Geometry: final body of the model. Coordinates: model frame, mm. A direction names the side the tool comes from. Coordinates: 2 decimals unless noted, no trailing zeros. Loops run counter-clockwise (first coordinate to the right, second up) from the corner with the lowest first, then second, coordinate; pieces in that order, holes last. Notation, with made-up numbers: (31.5, 60.25) - (48.5, 60.25) arc R26 cw to (48.5, 83.25) - close; hole circle Ø3 at (76.25, 9.5). An arc over 180 degrees is marked (long way). Return JSON: item names as keys, results as strings.
from build123d import *

# Parameters (mm, degrees)
F0_W      = 5
F0_H      = 25.21445
F1_DEPTH  = 25
F2_DEPTH  = 25
F3_W      = 40.349028
F3_H      = 25.21445
F3_W_2    = 5
F4_DEPTH  = 25
F6_DEPTH  = 25
F7_W      = 19.362385
F7_H      = 69.068812
F8_DEPTH  = 22
F9_W      = 17.915649
F9_H      = 21.240922
F10_DEPTH = 40


with BuildPart() as f1:
    # F0 (on Front) → F1 (new body)
    with BuildSketch(Plane.XZ):
        Polygon((0, 50.428901), (0, 25.21445), (5, 25.21445), (5, 45.428901), (50.775229, 45.428901), (50.775229, 0), (55.775229, 0), (55.775229, 50.428901), align=None)
        with Locations((2.5, 12.607225)):
            Rectangle(F0_W, F0_H)
    extrude(amount=-F1_DEPTH)

    # F0 (on Front) → F2 (join)
    with BuildSketch(Plane.XZ):
        with Locations((2.5, 12.607225)):
            Rectangle(F0_W, F0_H)
    extrude(amount=F2_DEPTH)

    # F3 (on face) → F4 (join)
    with BuildSketch(Plane.XZ.offset(25)):
        with Locations((25.174514, 12.607225)):
            Rectangle(F3_W, F3_H)
        with Locations((2.5, 12.607225)):
            Rectangle(F3_W_2, F3_H)
    extrude(amount=F4_DEPTH)

    # F5 (on face) → F6 (join)
    with BuildSketch(Plane(origin=(0, 0, 0), x_dir=(0, -1, 0), z_dir=(-1, 0, 0))):
        Polygon((-25, 25.21445), (-25, 0), (50, 0), (50, 25.21445), (0, 25.21445), align=None)
    extrude(amount=F6_DEPTH)

    # F7 (on face) → F8 (cut)
    with BuildSketch(Plane.XY.offset(25.21445)):
        with Locations((-12.571103, -12.137614)):
            Rectangle(F7_W, F7_H)
    extrude(amount=-F8_DEPTH, mode=Mode.SUBTRACT)

    # F9 (on face) → F10 (cut)
    with BuildSketch(Plane.YZ.offset(45.349028)):
        with Locations((-38.147681, 10.620461)):
            Rectangle(F9_W, F9_H)
    extrude(amount=-F10_DEPTH, mode=Mode.SUBTRACT)


solid = f1.part
Item 1: Section query A-A, the plane z = 23.5. Return loops of the section in (x, y).
Worked out:
{"outline": "(-25, -50) - (45.35, -50) - (45.35, -25) - (5, -25) - (5, 25) - (-25, 25) - close; (50.78, 0) - (55.78, 0) - (55.78, 25) - (50.78, 25) - close; hole (-22.25, -46.67) - (-2.89, -46.67) - (-2.89, 22.4) - (-22.25, 22.4) - close"}
Item 2: Mould query, pull axis Y, two halves, no side actions, for faces 1 (the face through (55.775, 12, 25)), 2 (the face through (26, -29.19, 10)), 3 (the face through (4, 25, 27)). Classes: +Y half, -Y half, draft (parallel to the pull), parting line (faces both ways), or undercut.
Worked out:
{"face 1": "draft", "face 2": "undercut", "face 3": "+Y half"}
Item 3: Section query D-D, the plane z = 35.5. Return loops of the section in (x, y).
Worked out:
{"outline": "(0, 0) - (5, 0) - (5, 25) - (0, 25) - close; (50.78, 0) - (55.78, 0) - (55.78, 25) - (50.78, 25) - close"}
Item 4: First-contact query: pin 1 Ø4 at (x, y) = (-10, -33) entering from +Z; pin 2 Ø19.5 at (y, z) = (-37, 10.5) entering from +X; pin 3 Ø20 at (x, y) = (21, 12.5) entering from -Z; pin 4 Ø1.5 at (x, y) = (47, -37) entering from +Z. Flat tips, straight axial feed; report the tip coordinate or a pass-through.
Worked out:
{"pin 1": "z = 3.21", "pin 2": "x = 45.35", "pin 3": "z = 45.43", "pin 4": "through"}
Item 5: Section query B-B, the plane x = 9. Return loops of the section in (y, z).
Worked out:
{"outline": "(-50, 0) - (-47.11, 0) - (-47.11, 21.24) - (-29.19, 21.24) - (-29.19, 0) - (-25, 0) - (-25, 25.21) - (-50, 25.21) - close; (0, 45.43) - (25, 45.43) - (25, 50.43) - (0, 50.43) - close"}
Item 6: Section query C-C, the plane y = -20.5. Return loops of the section in (x, z).
Worked out:
{"outline": "(-25, 0) - (5, 0) - (5, 25.21) - (-2.89, 25.21) - (-2.89, 3.21) - (-22.25, 3.21) - (-22.25, 25.21) - (-25, 25.21) - close"}
Item 7: Ray query, probe 1 along X at (y, z) = (-31, 19); probe 2 along X at (y, z) = (20.5, 10); probe 3 along Y at (x, z) = (33, 13.5). Return the intervals inside material, ascending. Write a range as from..to.
Worked out:
{"probe 1": "-25..-22.25, -2.89..5.35", "probe 2": "-25..-22.25, -2.89..5, 50.78..55.78", "probe 3": "-50..-47.11, -29.19..-25"}
Item 8: Reachability of faces 4 (the face through (32, 0, 46)), 5 (the face through (5.349, -38, 11)), 6 (the face through (-2.89, -13, 14)) from +Z, -Z, +X, -X, +Y, -Y: full face, straight path, thin tool, end or side. Return the list, or none.
Worked out:
{"face 4": "+Z, +X, -Y", "face 5": "-Z, +X", "face 6": "+Z"}
